from build123d import *

# Parameters (mm, degrees)
SKETCH1_R           = 50
BOSS_EXTRUDE1_DEPTH = 4
CUT_EXTRUDE1_DEPTH  = 12
SKETCH5_R           = 1.5
CUT_EXTRUDE2_DEPTH  = 4


with BuildPart() as part:
    # Sketch1 → Boss-Extrude1 (new body)
    with BuildSketch(Plane.XY):
        with Locations((-42.286719292, 29.938997259)):
            Circle(SKETCH1_R)
    extrude(amount=BOSS_EXTRUDE1_DEPTH)

    # Sketch4 → Cut-Extrude1 (cut)
    with BuildSketch(Plane.XY.offset(4)):
        Polygon((-42.286719292, 23.010794029), (-36.286719292, 26.474895644), (-36.286719292, 33.403098874), (-42.286719292, 36.867200489), (-48.286719292, 33.403098874), (-48.286719292, 26.474895644), align=None)
    extrude(amount=-CUT_EXTRUDE1_DEPTH, mode=Mode.SUBTRACT)

    # Sketch5 → Cut-Extrude2 (cut)
    with BuildSketch(Plane.XY.offset(4)):
        with Locations((-67.286719292, 29.938997259)):
            Circle(SKETCH5_R)
        with Locations((-42.286719292, 54.938997259)):
            Circle(SKETCH5_R)
        with Locations((-17.286719292, 29.938997259)):
            Circle(SKETCH5_R)
        with Locations((-42.286719292, 4.938997259)):
            Circle(SKETCH5_R)
    extrude(amount=-CUT_EXTRUDE2_DEPTH, mode=Mode.SUBTRACT)


solid = part.part
Source: CAD feature listing. Evaluate the final solid. Frame: model axes, mm. A direction names the side the tool comes from. Coordinates: 2 decimals unless noted, no trailing zeros. Order: outer loops, then holes, each group sorted by start corner. A loop starts at its lowest first (then second) coordinate and runs counter-clockwise, first axis right, second up.
Item 1: Cut plane B-B (z = 0.95). Return loops of the section in (x, y).
Output values:
outline: circle Ø100 at (-42.29, 29.94); hole circle Ø3 at (-67.29, 29.94); hole (-48.29, 26.47) - (-42.29, 23.01) - (-36.29, 26.47) - (-36.29, 33.4) - (-42.29, 36.87) - (-48.29, 33.4) - close; hole circle Ø3 at (-42.29, 4.94); hole circle Ø3 at (-42.29, 54.94); hole circle Ø3 at (-17.29, 29.94)
Item 2: Pull-direction query (X, two-part tool) for faces 1 (the face through (-40.901, 54.364, 2.028)), 2 (the face through (-48.287, 30, 2)), 3 (the face through (-48.796, 79.514, 1.972)), 4 (the face through (-43, 20, 0)); classes: pulls with the +X half, pulls with the -X half, needs draft (parallel to the pull), parting line crosses it, or undercut.
Output values:
face 1: undercut
face 2: undercut
face 3: parting line crosses it
face 4: needs draft
Item 3: Set-up query: faces 5 (the face through (-45.24, 35.16, 2.03)), 6 (the face through (-43, 20, 4)). Return all of +Z, -Z, +X, -X, +Y, -Y with unobstructed straight access to the full face (end or side cutting, diameter ignored); none if empty.
Output values:
face 5: +Z, -Z
face 6: +Z, +X, -X, +Y, -Y
Item 4: First-contact query: P1, Ø6, axis at x = -49.5, y = 46, coming from the -Z side; P2, Ø2, axis at y = 48, z = 1, coming from the +X side; P3, Ø1.5, axis at x = -73, z = 2, coming from the +Y side; P4, Ø1, axis at x = -40.5, z = 1, coming from the -Y side. Flat tips, straight axial feed; report the tip coordinate or a pass-through.
Output values:
P1: stops at z = 0
P2: stops at x = 4.71
P3: stops at y = 69.97
P4: stops at y = -20.04
Item 5: Cut plane C-C (x = -61). Return loops of the section in (y, z), plus the area to 3 significant figures.
Output values:
outline: (-16.43, 0) - (76.31, 0) - (76.31, 4) - (-16.43, 4) - close
area: 371 mm2
Item 6: Cut plane D-D (y = 0). Return loops of the section in (x, z), plus the area to 3 significant figures.
Output values:
outline: (-82.33, 0) - (-2.24, 0) - (-2.24, 4) - (-82.33, 4) - close
area: 320 mm2
Item 7: Cut plane A-A (y = 24.5). Return loops of the section in (x, z).
Output values:
outline: (-91.99, 0) - (-44.87, 0) - (-44.87, 4) - (-91.99, 4) - close; (-39.71, 0) - (7.42, 0) - (7.42, 4) - (-39.71, 4) - close
Item 8: Material intervals for line 1 (Y direction, x = -44.5, z = 0.35); line 2 (X direction, y = 24.5, z = 1); line 3 (X direction, y = 26.5, z = 2.2), sorted ascending.
Output values:
line 1: y = -20.01 to 24.29, 35.59 to 79.89
line 2: x = -91.99 to -44.87, -39.71 to 7.42
line 3: x = -92.17 to -48.29, -36.29 to 7.59
